Build history of the part. All positions in model axes, mm. A direction names the side the tool comes from. Give positions to 0.01 mm unless a question says otherwise; leave off trailing zeros. Order: outer loops, then holes, each group sorted by start corner. A loop starts at its lowest first (then second) coordinate and runs counter-clockwise, first axis right, second up. Notation, with made-up numbers: (23.5, 39.5) - (66.5, 39.5) arc R32 cw to (66.5, 71.5) - close; hole circle Ø11 at (-22, 85). An arc over 180 degrees is marked (long way). Answer in a Markdown table with one row per item.
```python
from build123d import *

# Parameters (mm, degrees)
F1_DEPTH = 5
F5_DEPTH = 7
F6_DEPTH = 7


with BuildPart() as f1:
    # F0 (on Top) → F1 (new body)
    with BuildSketch(Plane.XY):
        with BuildLine():
            Line((20.5, 0), (0, 0))
            Line((0, 0), (0, 5.2))
            Line((0, 5.2), (1.8, 5.2))
            Line((1.8, 5.2), (0.502887, 8.942781))
            ThreePointArc((0.502887, 8.942781), (-0.232808, 9.856134), (-1.354066, 10.2))
            Line((-1.354066, 10.2), (-3, 10.2))
            ThreePointArc((-3, 10.2), (-4.414214, 9.614214), (-5, 8.2))
            Line((-5, 8.2), (-5, -3))
            ThreePointArc((-5, -3), (-4.414214, -4.414214), (-3, -5))
            Line((-3, -5), (23.5, -5))
            ThreePointArc((23.5, -5), (24.914214, -4.414214), (25.5, -3))
            Line((25.5, -3), (25.5, 0))
            Line((25.5, 0), (25.5, 8.2))
            ThreePointArc((25.5, 8.2), (24.914214, 9.614214), (23.5, 10.2))
            Line((23.5, 10.2), (21.854066, 10.2))
            ThreePointArc((21.854066, 10.2), (20.732808, 9.856134), (19.997113, 8.942781))
            Line((19.997113, 8.942781), (18.7, 5.2))
            Line((18.7, 5.2), (20.5, 5.2))
            Line((20.5, 5.2), (20.5, 0))
        make_face()
    extrude(amount=F1_DEPTH)

    # F4 (on offset) → F5 (join)
    with BuildSketch(Plane.YZ.offset(10)):
        with BuildLine():
            ThreePointArc((-22.701302, 10.393598), (-23.433626, 10.642174), (-24.124238, 10.294118))
            ThreePointArc((-24.124238, 10.294118), (-20.645043, -8.08931), (-3.443092, -0.730769))
            ThreePointArc((-3.443092, -0.730769), (-3.084486, -0.203372), (-2.480016, 0))
            Line((-2.480016, 0), (0, 0))
            Line((0, 0), (0, 5))
            Line((0, 5), (-2.480016, 5))
            ThreePointArc((-2.480016, 5), (-3.084486, 5.203372), (-3.443092, 5.730769))
            ThreePointArc((-3.443092, 5.730769), (-3.739036, 6.646167), (-4.107359, 7.534916))
            ThreePointArc((-4.107359, 7.534916), (-4.680832, 8.057825), (-5.455624, 8.01307))
            Line((-5.455624, 8.01307), (-6.111157, 7.691379))
            ThreePointArc((-6.111157, 7.691379), (-6.612821, 7.128674), (-6.579024, 6.375572))
            ThreePointArc((-6.579024, 6.375572), (-16.267771, -6.6829), (-22.055883, 8.512273))
            ThreePointArc((-22.055883, 8.512273), (-21.819513, 9.231201), (-22.154452, 9.909835))
            Line((-22.154452, 9.909835), (-22.701302, 10.393598))
        make_face()
    extrude(amount=-F5_DEPTH)

    # F4 (on offset) → F6 (join)
    with BuildSketch(Plane.YZ.offset(10)):
        with BuildLine():
            ThreePointArc((-22.701302, 10.393598), (-23.433626, 10.642174), (-24.124238, 10.294118))
            ThreePointArc((-24.124238, 10.294118), (-20.645043, -8.08931), (-3.443092, -0.730769))
            ThreePointArc((-3.443092, -0.730769), (-3.084486, -0.203372), (-2.480016, 0))
            Line((-2.480016, 0), (0, 0))
            Line((0, 0), (0, 5))
            Line((0, 5), (-2.480016, 5))
            ThreePointArc((-2.480016, 5), (-3.084486, 5.203372), (-3.443092, 5.730769))
            ThreePointArc((-3.443092, 5.730769), (-3.739036, 6.646167), (-4.107359, 7.534916))
            ThreePointArc((-4.107359, 7.534916), (-4.680832, 8.057825), (-5.455624, 8.01307))
            Line((-5.455624, 8.01307), (-6.111157, 7.691379))
            ThreePointArc((-6.111157, 7.691379), (-6.612821, 7.128674), (-6.579024, 6.375572))
            ThreePointArc((-6.579024, 6.375572), (-16.267771, -6.6829), (-22.055883, 8.512273))
            ThreePointArc((-22.055883, 8.512273), (-21.819513, 9.231201), (-22.154452, 9.909835))
            Line((-22.154452, 9.909835), (-22.701302, 10.393598))
        make_face()
    extrude(amount=F6_DEPTH)


solid = f1.part
```
1. Cut at C-C on x = 23. Write the cut outline in (y, z), and give its area (3 significant figures).
Check result:
| item | result |
|---|---|
| outline | (-5, 0) - (10.2, 0) - (10.2, 5) - (-5, 5) - close |
| area | 76.0 mm² |
2. Drop flat-ended pins along their axis: P1, Ø16.5, axis at x = 6.5, y = 0, coming from the +Z side; P2, Ø1.5, axis at x = 3, y = -9, coming from the -Z side; P3, Ø0.9, axis at x = 1.5, z = 2, coming from the -Y side. Give the stop position or say it passes through.
Check result:
| item | result |
|---|---|
| P1 | stops at z = 8.12 |
| P2 | stops at z = -8.29 |
| P3 | stops at y = -5 |
3. Which spindle directions (+Z, -Z, +X, -X, +Y, -Y) get a long thin tool onto all of the face, cutting with end or side? Do faces 1 (the face through (20, -5, 2)), 2 (the face through (0, -5, 2)), 3 (the face through (19.36, 7.1, 2.46)). Say none if no direction does.
Check result:
| item | result |
|---|---|
| face 1 | +Z, -Z, +X, -Y |
| face 2 | +Z, -Z, -X, -Y |
| face 3 | +Z, -Z, +Y |
4. Cut at B-B on y = -23.5. Write the cut outline in (x, z), and give its area (3 significant figures).
Check result:
| item | result |
|---|---|
| outline | (3, -5.97) - (17, -5.97) - (17, -1.2) - (3, -1.2) - close; (3, 6.2) - (17, 6.2) - (17, 10.64) - (3, 10.64) - close |
| area | 129 mm² |
5. Cut at A-A on z = 2.5. Write the cut outline in (x, y), and give its area (3 significant figures).
Check result:
| item | result |
|---|---|
| outline | (-5, -3) arc R2 ccw to (-3, -5) - (3, -5) - (3, -5.73) - (17, -5.73) - (17, -5) - (23.5, -5) arc R2 ccw to (25.5, -3) - (25.5, 8.2) arc R2 ccw to (23.5, 10.2) - (21.85, 10.2) arc R2 ccw to (20, 8.94) - (18.7, 5.2) - (20.5, 5.2) - (20.5, 0) - (0, 0) - (0, 5.2) - (1.8, 5.2) - (0.5, 8.94) arc R2 ccw to (-1.35, 10.2) - (-3, 10.2) arc R2 ccw to (-5, 8.2) - close; (3, -27) - (17, -27) - (17, -24.27) - (3, -24.27) - close |
| area | 308 mm² |
6. Cut at D-D on z = -2. Write the cut outline in (x, y).
Check result:
| item | result |
|---|---|
| outline | (3, -26.12) - (17, -26.12) - (17, -23.1) - (3, -23.1) - close; (3, -6.9) - (17, -6.9) - (17, -3.88) - (3, -3.88) - close |
7. Two-plate mould, pull along Y, no slides. Class faces 4 (the face through (17, -19.3, -6.1)), 5 (the face through (-4.4, 9.63, 2.46)), 6 (the face through (0, 3, 2)): +Y half, -Y half, draft (parallel to the pull), parting line (faces both ways), or undercut.
Check result:
| item | result |
|---|---|
| face 4 | draft |
| face 5 | +Y half |
| face 6 | undercut |
8. Probe line 1 (Y direction, x = 11.5, z = 2.5); line 2 (X direction, y = 2.5, z = 2.75); line 3 (Z direction, x = 10.75, y = -15). List the from-to ranges inside material, lowest first.
Check result:
| item | result |
|---|---|
| line 1 | y = -27 to -24.27, -5.73 to 0 |
| line 2 | x = -5 to 0, 20.5 to 25.5 |
| line 3 | z = -9.5 to -6.77 |
